The listing builds one solid part. Answer for the finished solid, in the listing's coordinates (mm). A direction names the side the tool comes from. Coordinates: 2 decimals unless noted, no trailing zeros. Write each loop counter-clockwise with the first axis right and the second up, starting at its lowest first coordinate (ties: lowest second). Pieces come first, ordered by that corner, then holes.
from build123d import *

# Parameters (mm, degrees)
REVOLVE1_ANGLE      = 180
BOSS_EXTRUDE4_START = -20
BOSS_EXTRUDE4_DEPTH = 20
CUT_EXTRUDE4_DEPTH  = 20
SKETCH12_W          = 16
SKETCH12_H          = 12
BOSS_EXTRUDE6_DEPTH = 16.5
SKETCH13_W          = 8
SKETCH13_H          = 4
CUT_EXTRUDE6_DEPTH  = 15
SKETCH14_R          = 2.75
CUT_EXTRUDE7_DEPTH  = 15


with BuildPart() as part:
    # Sketch1 → Revolve1 (revolve)
    with BuildSketch(Plane(origin=(0, 0, 0), x_dir=(1, 0, 0), z_dir=(0, 1, 0))):
        Polygon((0, 0), (0, 7), (-2, 7), (-2, 13), (0, 13), (0, 17), (-2, 17), (-2, 20), (4, 20), (4, 17), (4, 0), align=None)
    revolve(axis=Axis((-8, 0, 0), (0, 0, -1)), revolution_arc=REVOLVE1_ANGLE)

    # Sketch8 → Boss-Extrude4 (add)
    with BuildSketch(Plane(origin=(0, 0, -20), x_dir=(-1, 0, 0), z_dir=(0, 0, -1)).offset(BOSS_EXTRUDE4_START)):
        with BuildLine():
            Line((20, 0), (35.5, 0))
            Line((35.5, 0), (35.5, -13.7))
            Line((35.5, -13.7), (-19.5, -13.7))
            Line((-19.5, -13.7), (-19.5, 0))
            Line((-19.5, 0), (-4, 0))
            ThreePointArc((-4, 0), (8, -12), (20, 0))
        make_face()
    extrude(amount=BOSS_EXTRUDE4_DEPTH)

    # Sketch9 → Cut-Extrude4 (cut)
    with BuildSketch(Plane(origin=(0, 0, 0), x_dir=(1, 0, 0), z_dir=(0, 1, 0))):
        with BuildLine():
            Line((-33, 5), (-33, 11))
            ThreePointArc((-33, 11), (-31, 13), (-29, 11))
            Line((-29, 11), (-29, 5))
            ThreePointArc((-29, 5), (-31, 3), (-33, 5))
        make_face()
        with BuildLine():
            Line((-19, 5), (-19, 11))
            ThreePointArc((-19, 11), (-21, 13), (-23, 11))
            Line((-23, 11), (-23, 5))
            ThreePointArc((-23, 5), (-21, 3), (-19, 5))
        make_face()
        with BuildLine():
            Line((3, 5), (3, 11))
            ThreePointArc((3, 11), (5, 13), (7, 11))
            Line((7, 11), (7, 5))
            ThreePointArc((7, 5), (5, 3), (3, 5))
        make_face()
        with BuildLine():
            Line((17, 5), (17, 11))
            ThreePointArc((17, 11), (15, 13), (13, 11))
            Line((13, 11), (13, 5))
            ThreePointArc((13, 5), (15, 3), (17, 5))
        make_face()
    extrude(amount=-CUT_EXTRUDE4_DEPTH, mode=Mode.SUBTRACT)

    # Sketch12 → Boss-Extrude6 (add)
    with BuildSketch(Plane(origin=(0, -13.7, 0), x_dir=(-1, 0, 0), z_dir=(0, -1, 0))):
        with Locations((8, 12)):
            Rectangle(SKETCH12_W, SKETCH12_H)
    extrude(amount=BOSS_EXTRUDE6_DEPTH)

    # Sketch13 → Cut-Extrude6 (cut)
    with BuildSketch(Plane(origin=(0, -30.2, 0), x_dir=(-1, 0, 0), z_dir=(0, -1, 0))):
        with Locations((8, 12)):
            Rectangle(SKETCH13_W, SKETCH13_H)
    extrude(amount=-CUT_EXTRUDE6_DEPTH, mode=Mode.SUBTRACT)

    # Sketch14 → Cut-Extrude7 (cut)
    with BuildSketch(Plane(origin=(0, 0, -18), x_dir=(-1, 0, 0), z_dir=(0, 0, -1))):
        with Locations((8, -23.95)):
            Circle(SKETCH14_R)
    extrude(amount=-CUT_EXTRUDE7_DEPTH, mode=Mode.SUBTRACT)


solid = part.part
Q1. The part is cut by section D-D, the plane z = -2.25. Write down the section's boundary in (x, y), then the cut area to 3 significant figures.
Answers below:
outline: (-35.5, -13.7) - (19.5, -13.7) - (19.5, 0) - (0, 0) arc R8 cw to (-16, 0) - (-35.5, 0) - close
area: 653 mm2
Q2. The part is cut by section B-B, the plane y = -23.95. Write down the section's boundary in (x, z).
Answers below:
outline: (-16, -18) - (-10.75, -18) - (-10.75, -14) - (-12, -14) - (-12, -10) - (-10.75, -10) - (-10.75, -6) - (-16, -6) - close; (-5.25, -18) - (0, -18) - (0, -6) - (-5.25, -6) - (-5.25, -10) - (-4, -10) - (-4, -14) - (-5.25, -14) - close
Q3. Which of the six approach directions +Z, -Z, +X, -X, +Y, -Y give full straight-line access (tool end or side, diameter ignored) to faces 5 (the face through (-8, -8, -4)), 6 (the face through (-8.4, -8.3, 0)), 7 (the face through (-9.27, -26.39, -16.03)), 8 (the face through (-33, -7, -8)), 9 (the face through (-12, -23, -12))?
Answers below:
face 5: +Z, +Y
face 6: +Z, +X, -X, +Y, -Y
face 7: +Z, -Z
face 8: +Y, -Y
face 9: -Y
Q4. The part is cut by section C-C, the plane x = -21. Write down the section's boundary in (y, z), then the cut area to 3 significant figures.
Answers below:
outline: (-13.7, -20) - (0, -20) - (0, -13) - (-13.7, -13) - close; (-13.7, -3) - (0, -3) - (0, 0) - (-13.7, 0) - close
area: 137 mm2
Q5. Determine the mould class of faces 1 (the face through (-31, -7, -13)), 2 (the face through (-23, -7, -8)), 3 (the face through (-8, -13.7, -5)), 4 (the face through (19.5, -7, -10)) for opening direction X: released by +X, released by -X, zero draft, split by the parting line, or undercut.
Answers below:
face 1: undercut
face 2: undercut
face 3: zero draft
face 4: released by +X
Q6. Find the intervals of material crossed by probe 1 along X at (y, z) = (-13, -9.5); probe 2 along Y at (x, z) = (-8, -8.85); probe 3 along X at (y, z) = (-4, -8.75), in increasing order.
Answers below:
probe 1: x = -35.5 to -33, -29 to -23, -19 to 3, 7 to 13, 17 to 19.5
probe 2: y = -30.2 to -26.7, -21.2 to -6
probe 3: x = -35.5 to -33, -29 to -23, -19 to -12.47, -3.53 to 3, 7 to 13, 17 to 19.5
Q7. Given pin 1 (8 mm diameter, centred on y = -19, z = -18, fed in from +X); pin 2 (8 mm diameter, centred on x = -7, y = -25.5, fed in from -Z); pin 3 (4.5 mm diameter, centred on y = -22, z = -11.5, fed in from -X), each flat-ended and moving along its own axis, determine where each tip first touches the part or whether it passes through.
Answers below:
pin 1: stops at x = 0
pin 2: stops at z = -18
pin 3: stops at x = -16
Q8. The part is cut by section A-A, the plane x = -8. Write down the section's boundary in (y, z).
Answers below:
outline: (-30.2, -18) - (-26.7, -18) - (-26.7, -14) - (-30.2, -14) - close; (-30.2, -10) - (-26.7, -10) - (-26.7, -6) - (-30.2, -6) - close; (-21.2, -18) - (-13.7, -18) - (-13.7, -20) - (-6, -20) - (-6, -17) - (-8, -17) - (-8, -13) - (-6, -13) - (-6, -7) - (-8, -7) - (-8, 0) - (-13.7, 0) - (-13.7, -6) - (-21.2, -6) - (-21.2, -10) - (-15.2, -10) - (-15.2, -14) - (-21.2, -14) - close
